from build123d import *

# Parameters (mm, degrees)
EXTRUDE_1_DEPTH     = 40
CUT_EXTRUDE_1_DEPTH = 40
SKETCH_4_R          = 2.5
CUT_EXTRUDE_2_DEPTH = 54.38539126
SKETCH_5_R          = 2.5
CUT_EXTRUDE_3_DEPTH = 54.38539126
FILLET_1_R          = 2


with BuildPart() as part:
    # 草图1 → 凸台-拉伸1 (new body)
    with BuildSketch(Plane(origin=(0, 0, 0), x_dir=(0, 0, -1), z_dir=(1, 0, 0))):
        Polygon((0, 0), (0, 25), (25, 25), (25, 0), (23, 0), (23, 23), (2, 23), (2, 0), align=None)
    extrude(amount=EXTRUDE_1_DEPTH)

    # 草图3 → 切除-拉伸1 (cut)
    with BuildSketch(Plane.XY):
        with BuildLine():
            Line((40, 25), (40, 0))
            Line((40, 0), (6.458980338, 0))
            ThreePointArc((6.458980338, 0), (27.375481001, 6.937569599), (40, 25))
        make_face()
    extrude(amount=-CUT_EXTRUDE_1_DEPTH, mode=Mode.SUBTRACT)

    # 草图4 → 切除-拉伸2 (cut, through all)
    with BuildSketch(Plane(origin=(0, 25, 0), x_dir=(1, 0, 0), z_dir=(0, 1, 0))):
        with Locations(Location((31, 15, 0), (0, 0, 270))):
            Circle(SKETCH_4_R)
    extrude(amount=-CUT_EXTRUDE_2_DEPTH, mode=Mode.SUBTRACT)

    # 草图5 → 切除-拉伸3 (cut, through all)
    with BuildSketch(Plane.XY):
        with Locations((5, 7)):
            Circle(SKETCH_5_R)
    extrude(amount=-CUT_EXTRUDE_3_DEPTH, mode=Mode.SUBTRACT)

    # 圆角1
    fillet_1_edges = [part.edges().sort_by_distance(p)[0] for p in [
        (20, 25, 0),
        (20, 25, -25),
        (19.668772392, 23, -23),
        (19.668772392, 23, -2),
    ]]
    fillet(fillet_1_edges, radius=FILLET_1_R)


solid = part.part
Check sheet for the modelled part. Datum: model origin and axes. Units: mm. A direction names the side the tool comes from. Round coordinates to 2 decimals unless told otherwise and drop trailing zeros. Write each loop counter-clockwise with the first axis right and the second up, starting at its lowest first coordinate (ties: lowest second). Pieces come first, ordered by that corner, then holes. Notation, with made-up numbers: (-26.75, -3) - (-1.75, -3) arc R31 ccw to (-1.75, 25) - close; hole circle Ø11 at (67, -7.75). An arc over 180 degrees is marked (long way). Return JSON: item names as keys, results as strings.
Q1. Cross-section at C-C (y = 7). Record the boundary of the cut face in (x, z).
Returned:
{"outline": "(0, -25) - (2.5, -25) - (2.5, -23) - (0, -23) - close; (0, -2) - (2.5, -2) - (2.5, 0) - (0, 0) - close; (7.5, -25) - (27.46, -25) - (27.46, -23) - (7.5, -23) - close; (7.5, -2) - (27.46, -2) - (27.46, 0) - (7.5, 0) - close"}
Q2. Access from +Z, -Z, +X, -X, +Y, -Y to the whole of each face (thin tool, end or side, straight path). Record for faces 5 (the flat face through (15, 13, -23)), 6 (the cylindrical face through (31.071, 10.115, -23.553)).
Returned:
{"face 5": "+X, -X, -Y", "face 6": "+Z, -Z, +X, -Y"}
Q3. Cross-section at B-B (x = 33). Record the boundary of the cut face in (y, z).
Returned:
{"outline": "(12.18, -25) - (23, -25) arc R2 ccw to (25, -23) - (25, -16.5) - (23, -16.5) - (23, -21) arc R2 cw to (21, -23) - (12.18, -23) - close; (12.18, -2) - (21, -2) arc R2 cw to (23, -4) - (23, -13.5) - (25, -13.5) - (25, -2) arc R2 ccw to (23, 0) - (12.18, 0) - close"}
Q4. Cross-section at A-A (x = 5). Record the boundary of the cut face in (y, z).
Returned:
{"outline": "(0, -25) - (4.5, -25) - (4.5, -23) - (0, -23) - close; (0, -2) - (4.5, -2) - (4.5, 0) - (0, 0) - close; (9.5, -25) - (23, -25) arc R2 ccw to (25, -23) - (25, -2) arc R2 ccw to (23, 0) - (9.5, 0) - (9.5, -2) - (21, -2) arc R2 cw to (23, -4) - (23, -21) arc R2 cw to (21, -23) - (9.5, -23) - close"}
Q5. Draft check along X on faces 1 (the flat face through (0, 24, -14)), 2 (the cylindrical face through (6.15, 4.78, -23.99)), 3 (the cylindrical face through (32.69, 24.01, -16.84)), 4 (the cylindrical face through (19.94, 22.43, -2.6)). Enter one of: released by +X, released by -X, zero draft, split by the parting line, or undercut.
Returned:
{"face 1": "released by -X", "face 2": "undercut", "face 3": "undercut", "face 4": "zero draft"}
Q6. Cross-section at D-D (y = 2.25). Record the boundary of the cut face in (x, z), then the cut area to 3 significant figures.
Returned:
{"outline": "(0, -25) - (18.81, -25) - (18.81, -23) - (0, -23) - close; (0, -2) - (18.81, -2) - (18.81, 0) - (0, 0) - close", "area": "75.2 mm²"}
Q7. Scan lines: L1, parallel to Z at x = 9, y = 10.25; L2, parallel to Y at x = 35, z = -5; L3, parallel to X at y = 23.4, z = -15. Record each from-to range of solid material in increasing order. Write a range as from..to.
Returned:
{"L1": "z = -25..-23, -2..0", "L2": "y = 23..25", "L3": "x = 0..28.5, 33.5..39.48"}
Q8. Depth check by flat-ended pin: P1, Ø5, axis at y = 3, z = -21.5, coming from the +X side; P2, Ø6, axis at x = 31, z = -15, coming from the -Y side. Enter the tip coordinate at first touch or a pass-through.
Returned:
{"P1": "stops at x = 24.49", "P2": "stops at y = 23"}
